Work out the finished part from the listing and answer in its coordinate system (mm). A direction names the side the tool comes from. Give positions to 0.01 mm unless a question says otherwise; leave off trailing zeros. Order: outer loops, then holes, each group sorted by start corner. A loop starts at its lowest first (then second) coordinate and runs counter-clockwise, first axis right, second up.
```python
from build123d import *

# Parameters (mm, degrees)
SKETCH_1_W      = 23
SKETCH_1_H      = 23
SKETCH_1_R      = 1.5
EXTRUDE_1_DEPTH = 1.5
SKETCH_2_W      = 5
SKETCH_2_H      = 8
EXTRUDE_2_DEPTH = 2


with BuildPart() as part:
    # 草图1 → 凸台-拉伸1 (new body)
    with BuildSketch(Plane(origin=(0, 0, 0), x_dir=(1, 0, 0), z_dir=(0, 1, 0))):
        Rectangle(SKETCH_1_W, SKETCH_1_H)
        with Locations(Location((8.5, 8.5, 0), (0, 0, 270))):
            Circle(SKETCH_1_R, mode=Mode.SUBTRACT)
        with Locations(Location((8.5, -8.5, 0), (0, 0, 90))):
            Circle(SKETCH_1_R, mode=Mode.SUBTRACT)
        with Locations(Location((-8.5, -8.5, 0), (0, 0, 270))):
            Circle(SKETCH_1_R, mode=Mode.SUBTRACT)
        with Locations(Location((-8.5, 8.5, 0), (0, 0, 90))):
            Circle(SKETCH_1_R, mode=Mode.SUBTRACT)
    extrude(amount=EXTRUDE_1_DEPTH)

    # 草图2 → 凸台-拉伸2 (add)
    with BuildSketch(Plane(origin=(0, 1.5, 0), x_dir=(1, 0, 0), z_dir=(0, 1, 0))):
        Rectangle(SKETCH_2_W, SKETCH_2_H)
    extrude(amount=EXTRUDE_2_DEPTH)


solid = part.part
```
1. Given P1, Ø5, axis at x = 8.5, z = -8.5, coming from the +Y side; P2, Ø2.5, axis at x = 8.5, z = 8.5, coming from the +Y side; P3, Ø12, axis at x = -7.5, z = -1, coming from the -Y side; P4, Ø1.6, axis at y = 3, z = 0, coming from the +X side, each flat-ended and moving along its own axis, determine where each tip first touches the part or whether it passes through.
Findings below:
P1: stops at y = 1.5
P2: passes through
P3: stops at y = 0
P4: stops at x = 2.5
2. The mould has two halves that part along X. Classify faces 6 (the face through (2.5, 2, 0)), 7 (the face through (0, 1, 11.5)), 8 (the face through (7.6, 0.7, -9.7)), 9 (the face through (-11.5, 1, 0)): pulls with the +X half, pulls with the -X half, needs draft (parallel to the pull), parting line crosses it, or undercut.
Findings below:
face 6: pulls with the +X half
face 7: needs draft
face 8: undercut
face 9: pulls with the -X half
3. Which of the six approach directions +Z, -Z, +X, -X, +Y, -Y give full straight-line access (tool end or side, diameter ignored) to faces 1 (the face through (0, 2, 4)), 2 (the face through (0, 3.5, 0)), 3 (the face through (0, 2, -4)), 4 (the face through (-2.5, 2, 0)), 5 (the face through (9.4, 0.7, 9.7))?
Findings below:
face 1: +Z, +X, -X, +Y
face 2: +Z, -Z, +X, -X, +Y
face 3: -Z, +X, -X, +Y
face 4: +Z, -Z, -X, +Y
face 5: +Y, -Y
4. The part is cut by section A-A (z = 8.5). Write down the section's boundary in (x, y), then the cut area to 3 significant figures.
Findings below:
outline: (-11.5, 0) - (-10, 0) - (-10, 1.5) - (-11.5, 1.5) - close; (-7, 0) - (7, 0) - (7, 1.5) - (-7, 1.5) - close; (10, 0) - (11.5, 0) - (11.5, 1.5) - (10, 1.5) - close
area: 25.5 mm2
5. The part is cut by section C-C (y = 0.75). Write down the section's boundary in (x, z).
Findings below:
outline: (-11.5, -11.5) - (11.5, -11.5) - (11.5, 11.5) - (-11.5, 11.5) - close; hole circle Ø3 at (-8.5, -8.5); hole circle Ø3 at (-8.5, 8.5); hole circle Ø3 at (8.5, -8.5); hole circle Ø3 at (8.5, 8.5)
6. The part is cut by section B-B (x = -8). Write down the section's boundary in (y, z), then the cut area to 3 significant figures.
Findings below:
outline: (0, -11.5) - (1.5, -11.5) - (1.5, -9.91) - (0, -9.91) - close; (0, -7.09) - (1.5, -7.09) - (1.5, 7.09) - (0, 7.09) - close; (0, 9.91) - (1.5, 9.91) - (1.5, 11.5) - (0, 11.5) - close
area: 26.0 mm2
7. Straight lines are drawn through the part: probe 1 along X at (y, z) = (1.2, -8.5); probe 2 along Y at (x, z) = (7.5, -6.5); probe 3 along Z at (x, y) = (2, 2.75). For each, find the intervals that lie inside material, in ascending order.
Findings below:
probe 1: x = -11.5 to -10, -7 to 7, 10 to 11.5
probe 2: y = 0 to 1.5
probe 3: z = -4 to 4
8. The part is cut by section D-D (x = 5.25). Write down the section's boundary in (y, z).
Findings below:
outline: (0, -11.5) - (1.5, -11.5) - (1.5, 11.5) - (0, 11.5) - close
